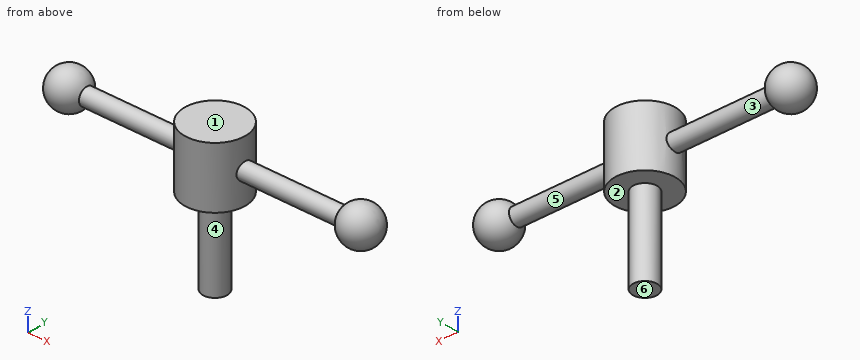
from build123d import *

# Parameters (mm, degrees)
F3_W     = 152.4
F3_H     = 4.445
F2_W     = 15.875
F2_H     = 31.75
F6_R     = 6.35
F7_DEPTH = 44.45


with BuildPart() as f1:
    # F0 (on Front) → F1 (revolve)
    with BuildSketch(Plane.XZ):
        with BuildLine():
            Line((-86.356572, 25.4), (-66.036572, 25.4))
            ThreePointArc((-66.036572, 25.4), (-76.196572, 35.56), (-86.356572, 25.4))
        make_face()
        with BuildLine():
            Line((66.043428, 25.4), (86.363428, 25.4))
            ThreePointArc((86.363428, 25.4), (76.203428, 35.56), (66.043428, 25.4))
        make_face()
    revolve(axis=Axis((-76.196572, 0, 25.4), (1, 0, 0)))

    # F3 (on Front) → F4 (revolve)
    with BuildSketch(Plane.XZ):
        with Locations((0, 27.6225)):
            Rectangle(F3_W, F3_H)
    revolve(axis=Axis((0, 0, 25.4), (1, 0, 0)))

    # F2 (on Front) → F5 (revolve)
    with BuildSketch(Plane.XZ):
        with Locations((7.9375, 25.4)):
            Rectangle(F2_W, F2_H)
    revolve(axis=Axis((0, 0, 25.4), (0, 0, -1)))

    # F6 (on face) → F7 (join)
    with BuildSketch(Plane(origin=(0, 0, 9.525), x_dir=(1, 0, 0), z_dir=(0, 0, -1))):
        Circle(F6_R)
    extrude(amount=F7_DEPTH)


solid = f1.part
Model file for the job. Use its own axes, mm. Face numbers are marked on the shaded views. A direction names the side the tool comes from. Give positions to 0.01 mm unless a question says otherwise; leave off trailing zeros. Loops run counter-clockwise (first coordinate to the right, second up) from the corner with the lowest first, then second, coordinate; pieces in that order, holes last.
1) Saw through at C-C (x = 0). Write the cut outline in (y, z) (3 decimals).
2) Flat gauge pins, fed straight in: pin 1 Ø3 at (y, z) = (-8.5, 1.5) entering from -X; pin 2 Ø10 at (y, z) = (-1, -7.5) entering from +X; pin 3 Ø4 at (x, z) = (5, 15.5) entering from +Y; pin 4 Ø1.5 at (y, z) = (-9, 27.5) entering from +X. Where does each tip first touch, or does it go through?
3) Wall check: line 1 (X direction, y = -0.5, z = 6); line 2 (X direction, y = 5.5, z = 26); line 3 (Z direction, x = -12.5, y = -7) (3 decimals). Give the ranges that are in metal, low to high.
4) Saw through at D-D (x = 31.5). Write the cut outline in (y, z) (3 decimals), plus the area to 3 significant figures.
5) Tool access for the marked faces 1 and 2: list every direction of +Z, -Z, +X, -X, +Y, -Y with a clear straight run to the whole face (end or side of a thin tool).
6) Saw through at A-A (y = 0). Write the cut outline in (x, z) (3 decimals).
7) Pull direction X, two halves, no side cores. Call the marked faces 3, 4, 5 and 6: +X half, -X half, draft (parallel to the pull), parting line (faces both ways), or undercut.
8) Saw through at B-B (z = 25.4). Write the cut outline in (x, y) (3 decimals), plus the area to 3 significant figures.
Answer block:
1. outline: (-15.875, 9.525) - (-6.35, 9.525) - (-6.35, -34.925) - (6.35, -34.925) - (6.35, 9.525) - (15.875, 9.525) - (15.875, 41.275) - (-15.875, 41.275) - close
2. pin 1: passes through
2. pin 2: stops at x = 6.35
2. pin 3: stops at y = 15.59
2. pin 4: stops at x = 81.78
3. line 1: x = -6.33 to 6.33
3. line 2: x = -84.72 to -67.68, -14.89 to 14.89, 67.68 to 84.72
3. line 3: z = 9.525 to 41.275
4. outline: circle Ø8.89 at (0, 25.4)
4. area: 62.1 mm2
5. face 1: +Z, +X, -X, +Y, -Y
5. face 2: -Z
6. outline: (-67.061, 20.955) - (-15.875, 20.955) - (-15.875, 9.525) - (-6.35, 9.525) - (-6.35, -34.925) - (6.35, -34.925) - (6.35, 9.525) - (15.875, 9.525) - (15.875, 20.955) - (67.067, 20.955) arc R10.16 ccw (long way) to (67.067, 29.845) - (15.875, 29.845) - (15.875, 41.275) - (-15.875, 41.275) - (-15.875, 29.845) - (-67.061, 29.845) arc R10.16 ccw (long way) to start
7. face 3: undercut
7. face 4: parting line
7. face 5: undercut
7. face 6: draft
8. outline: (-67.061, -4.445) - (-15.24, -4.445) arc R15.875 ccw to (15.24, -4.445) - (67.067, -4.445) arc R10.16 ccw (long way) to (67.067, 4.445) - (15.24, 4.445) arc R15.875 ccw to (-15.24, 4.445) - (-67.061, 4.445) arc R10.16 ccw (long way) to start
8. area: 2,340 mm2
